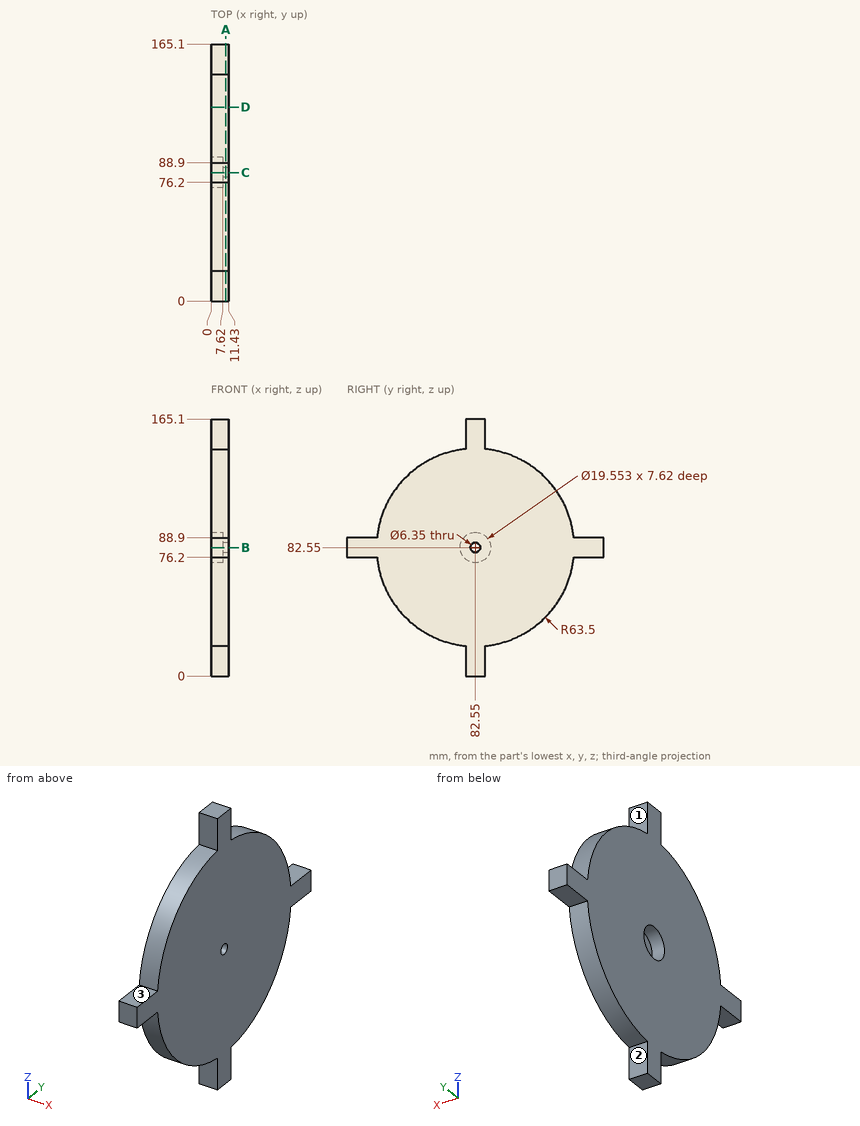
Check sheet for the drawn part. Datum: minimum x, y, z corner. Units: mm. A direction names the side the tool comes from. Round coordinates to 2 decimals unless told otherwise and drop trailing zeros. Order: outer loops, then holes, each group sorted by start corner. A loop starts at its lowest first (then second) coordinate and runs counter-clockwise, first axis right, second up. Notation, with made-up numbers: (-21.5, -15) -> (25.5, -15) arc R12 ccw to (25.5, -10) -> close; hole circle Ø4 at (65.25, 35). An arc over 180 degrees is marked (long way). Return JSON: item names as keys, results as strings. Group by question number.
Q1. Section check D-D, the plane y = 124.5. Record the boundary of the cut face in (x, z).
Q2. Section check B-B, the plane z = 82.55. Record the boundary of the cut face in (x, y) (1 decimal), plus the area to 3 significant figures.
Q3. Material ranges on probe 1 along Y at (x, z) = (8.7, 82.55) (3 decimals); probe 2 along Y at (x, z) = (5, 82.55), recorded low to high. Write a range as from..to.
Q4. Section check A-A, the plane x = 9.5. Record the boundary of the cut face in (y, z) (3 decimals).
Q5. Gauge pin test, flat ends, axial feed: pin 1 (12 mm diameter, centred on y = 145, z = 104, fed in from -X); pin 2 (5 mm diameter, centred on x = 3, z = 21.5, fed in from +Y); pin 3 (5 mm diameter, centred on x = 3, y = 96.5, fed in from -Z); pin 4 (4 mm diameter, centred on x = 4.5, y = 143.5, fed in from -Z). Record the tip position at first contact, or that the pin passes through.
Q6. Tool access check on the marked faces 1, 2 and 3. Record the directions out of +Z, -Z, +X, -X, +Y, -Y that give a thin tool (end or side, any length) a straight path to the whole face; none if there is none.
Numbers:
{
 "1": {"outline": "(0, 34.88) -> (11.43, 34.88) -> (11.43, 130.22) -> (0, 130.22) -> close"},
 "2": {"outline": "(0, 0) -> (11.4, 0) -> (11.4, 79.4) -> (7.6, 79.4) -> (7.6, 72.8) -> (0, 72.8) -> close; (0, 92.3) -> (7.6, 92.3) -> (7.6, 85.7) -> (11.4, 85.7) -> (11.4, 165.1) -> (0, 165.1) -> close", "area": "1,710 mm^2"},
 "3": {"probe 1": "0..79.375, 85.725..165.1", "probe 2": "0..72.77, 92.33..165.1"},
 "4": {"outline": "(0, 76.2) -> (19.368, 76.2) arc R63.5 ccw to (76.2, 19.368) -> (76.2, 0) -> (88.9, 0) -> (88.9, 19.368) arc R63.5 ccw to (145.732, 76.2) -> (165.1, 76.2) -> (165.1, 88.9) -> (145.732, 88.9) arc R63.5 ccw to (88.9, 145.732) -> (88.9, 165.1) -> (76.2, 165.1) -> (76.2, 145.732) arc R63.5 ccw to (19.368, 88.9) -> (0, 88.9) -> close; hole circle Ø6.35 at (82.55, 82.55)"},
 "5": {"pin 1": "x = 0", "pin 2": "y = 107.13", "pin 3": "z = 20.09", "pin 4": "z = 58.95"},
 "6": {"face 1": "+Z, +X, -X, +Y", "face 2": "-Z, +X, -X, +Y", "face 3": "+Z, +X, -X, -Y"}
}
